The model under review builds one solid part; all positions refer to its coordinate system, in mm. A direction names the side the tool comes from. Coordinates: 2 decimals unless noted, no trailing zeros. Write each loop counter-clockwise with the first axis right and the second up, starting at its lowest first coordinate (ties: lowest second). Pieces come first, ordered by that corner, then holes. Notation, with made-up numbers: (51.25, -22) -> (57.25, -22) arc R12 cw to (57.25, -13) -> close; hole circle Ø2 at (30, 65). An arc over 180 degrees is marked (long way). Write each question's results on one line, items separated by ' | '.
```python
from build123d import *

# Parameters (mm, degrees)
F1_DEPTH   = 5
F4_D       = 3
F4_ON_F3_D = 3
F5_ANGLE   = 90


with BuildPart() as f1:
    # F0 (on Right) → F1 (new body, symmetric)
    with BuildSketch(Plane.YZ):
        with BuildLine():
            Line((3, 30), (0, 30))
            Line((0, 30), (0, 0))
            Line((0, 0), (30, 0))
            Line((30, 0), (30, 3))
            Line((30, 3), (7, 3))
            ThreePointArc((7, 3), (4.1715728753, 4.1715728753), (3, 7))
            Line((3, 7), (3, 30))
        make_face()
    extrude(amount=F1_DEPTH, both=True)

    # F4 (through all)
    with Locations(Plane.XY.offset(3)):
        with Locations((0, 25), (0, 10)):
            Hole(F4_D / 2)

    # F4 on F3 (through all)
    with Locations(Plane(origin=(0, 3, 0), x_dir=(-1, 0, 0), z_dir=(0, 1, 0))):
        with Locations((0, 25), (0, 10)):
            Hole(F4_ON_F3_D / 2)


with BuildPart() as f1_1:
    # F5: moved
    add(f1.part.rotate(Axis((5, 15, 0), (0, 1, 0)), F5_ANGLE))


solid = f1_1.part
```
Q1. Machinability: for faces 5 (the cylindrical face through (6.48, 8.67, 5.69)), 6 (the flat face through (23, 3, 5)), which of the approach directions +Z, -Z, +X, -X, +Y, -Y give a long, thin tool a straight path to every point of the face, cutting with its end or side? Answer none if there is none.
Solution:
face 5: +X, -X | face 6: +Z, -Z, +X, +Y
Q2. Clearance check with flat-ended pins moving along their axes: P1, Ø1, axis at x = 22, z = 8.5, coming from the +Y side; P2, Ø5, axis at y = 25, z = 5, coming from the +X side; P3, Ø8, axis at x = 24, y = 5, coming from the +Z side. State where each tip first meets the part, or that it passes through.
Solution:
P1: y = 3 | P2: x = 8 | P3: z = 10
Q3. Add section A-A (z = 5). Write out the cut boundary in (x, y).
Solution:
outline: (5, 0) -> (13.5, 0) -> (13.5, 3) -> (12, 3) arc R4 cw to (8, 7) -> (8, 8.5) -> (5, 8.5) -> close; (5, 11.5) -> (8, 11.5) -> (8, 23.5) -> (5, 23.5) -> close; (5, 26.5) -> (8, 26.5) -> (8, 30) -> (5, 30) -> close; (16.5, 0) -> (28.5, 0) -> (28.5, 3) -> (16.5, 3) -> close; (31.5, 0) -> (35, 0) -> (35, 3) -> (31.5, 3) -> close
Q4. Add section D-D (z = 7). Write out the cut boundary in (x, y).
Solution:
outline: (5, 0) -> (35, 0) -> (35, 3) -> (12, 3) arc R4 cw to (8, 7) -> (8, 30) -> (5, 30) -> close
Q5. Add section C-C (y = 25.75). Write out the cut boundary in (x, z).
Solution:
outline: (5, 0) -> (8, 0) -> (8, 3.7) -> (5, 3.7) -> close; (5, 6.3) -> (8, 6.3) -> (8, 10) -> (5, 10) -> close
Q6. Draft analysis for pull direction Z (two halves, no side actions). For faces 1 (the cylindrical face through (16.01, 1.48, 6.11)), 2 (the flat face through (20, 0, 5)), 3 (the flat face through (13.4, 2.7, 10)), 4 (the cylindrical face through (31.01, 1.48, 6.11)), state which applies: pulls with the +Z half, pulls with the -Z half, needs draft (parallel to the pull), parting line crosses it, or undercut.
Solution:
face 1: undercut | face 2: needs draft | face 3: pulls with the +Z half | face 4: undercut
Q7. For line 1 (Y direction, x = 5.9, z = 5); line 2 (X direction, y = 1.25, z = 5); line 3 (X direction, y = 28.75, z = 3.75), list the stretches that pass through material, from the lowest coordinate up. Write a range as from..to.
Solution:
line 1: 0..8.5, 11.5..23.5, 26.5..30 | line 2: 5..13.5, 16.5..28.5, 31.5..35 | line 3: 5..8
Q8. Add section B-B (x = 15). Write out the cut boundary in (y, z), plus the area to 3 significant figures.
Solution:
outline: (0, 0) -> (3, 0) -> (3, 3.5) -> (0, 3.5) -> close; (0, 6.5) -> (3, 6.5) -> (3, 10) -> (0, 10) -> close | area: 21.0 mm²
